from build123d import *

# Parameters (mm, degrees)
SKETCH1_W             = 156
SKETCH1_H             = 136
BOSS_EXTRUDE1_DEPTH   = 19.05
SKETCH2_W             = 37.5
SKETCH2_H             = 37.5
CUT_EXTRUDE1_DEPTH    = 106.218356288
SKETCH3_W             = 22.8
SKETCH3_H             = 12.5
CUT_EXTRUDE2_DEPTH    = 106.218356288
FILLET1_R             = 1
BOSS_EXTRUDE2_START   = -4.5
BOSS_EXTRUDE2_DEPTH   = 51.5
BOSS_EXTRUDE2_2_DEPTH = 3
BOSS_EXTRUDE2_START_2 = 44
BOSS_EXTRUDE2_3_DEPTH = 3
CUT_EXTRUDE3_REACH    = 130.365
SKETCH5_W             = 45.5
SKETCH5_H             = 6.35


# Read off the part's stored shape, not the designer's step: Boss-Extrude2
with BuildPart() as part:
    # Sketch1 → Boss-Extrude1 (new body)
    with BuildSketch(Plane(origin=(0, 0, 0), x_dir=(1, 0, 0), z_dir=(0, 1, 0))):
        Rectangle(SKETCH1_W, SKETCH1_H)
    extrude(amount=BOSS_EXTRUDE1_DEPTH)

    # Sketch2 → Cut-Extrude1 (cut, through all)
    with BuildSketch(Plane(origin=(0, 19.05, 0), x_dir=(1, 0, 0), z_dir=(0, 1, 0))):
        with Locations((32.5, -21.25)):
            Rectangle(SKETCH2_W, SKETCH2_H)
    extrude(amount=-CUT_EXTRUDE1_DEPTH, mode=Mode.SUBTRACT)

    # Sketch3 → Cut-Extrude2 (cut, through all)
    with BuildSketch(Plane(origin=(0, 19.05, 0), x_dir=(1, 0, 0), z_dir=(0, 1, 0))):
        with Locations((-32.65, -21.25)):
            Rectangle(SKETCH3_W, SKETCH3_H)
    extrude(amount=-CUT_EXTRUDE2_DEPTH, mode=Mode.SUBTRACT)

    # Fillet1
    fillet1_edges = [part.edges().sort_by_distance(p)[0] for p in [
        (-44.05, 19.05, 21.25),
        (-21.25, 19.05, 21.25),
    ]]
    fillet(fillet1_edges, radius=FILLET1_R)

    # Boss-Extrude2 outline → Boss-Extrude2 (add)
    with BuildSketch(Plane.XY.offset(BOSS_EXTRUDE2_START)):
        Polygon((-3, 19.05), (0, 19.05), (0, 73.655885813), (-3, 75.957866777), align=None)
    extrude(amount=BOSS_EXTRUDE2_DEPTH)

    # Boss-Extrude2 2 outline → Boss-Extrude2 2 (add)
    with BuildSketch(Plane.XY.offset(BOSS_EXTRUDE2_START)):
        Polygon((0, 73.655885813), (0, 19.05), (71.163775898, 19.05), align=None)
    extrude(amount=BOSS_EXTRUDE2_2_DEPTH)

    # Boss-Extrude2 3 outline → Boss-Extrude2 3 (add)
    with BuildSketch(Plane.XY.offset(BOSS_EXTRUDE2_START_2)):
        Polygon((0, 73.655885813), (0, 19.05), (71.163775898, 19.05), align=None)
    extrude(amount=BOSS_EXTRUDE2_3_DEPTH)

    # Sketch5 → Cut-Extrude3 (cut, up to next)
    with BuildSketch(Plane(origin=(0, 0, 0), x_dir=(0, 0, -1), z_dir=(1, 0, 0)), mode=Mode.PRIVATE) as cut_extrude3_sk1:
        with Locations((-21.25, 22.225)):
            Rectangle(SKETCH5_W, SKETCH5_H)
    cut_extrude3_tool1 = extrude(cut_extrude3_sk1.sketch, amount=-CUT_EXTRUDE3_REACH, mode=Mode.PRIVATE) & part.part
    add(cut_extrude3_tool1.solids().sort_by_distance((0, 22.225, 21.25))[0], mode=Mode.SUBTRACT)


solid = part.part
Input: part model. Units: mm. Frame: model coordinates. A direction names the side the tool comes from. Coordinates: 2 decimals unless noted, no trailing zeros. Loops run counter-clockwise (first coordinate to the right, second up) from the corner with the lowest first, then second, coordinate; pieces in that order, holes last. Notation, with made-up numbers: (-40, 44.25) -> (-14, 44.25) arc R19 ccw to (-14, 67.25) -> close; hole circle Ø4 at (41, 23). An arc over 180 degrees is marked (long way). One line per item, written item: value.
(1) Set-up query: faces 5 (the face through (-1, 9, 68)), 6 (the face through (17, 35, 47)), 7 (the face through (-3, 48, 21)), 8 (the face through (32, 10, 2.5)), 9 (the face through (17, 35, -4.5)). Return all of +Z, -Z, +X, -X, +Y, -Y with unobstructed straight access to the full face (end or side cutting, diameter ignored); none if empty.
Answer below:
face 5: +Z, +X, -X, +Y, -Y
face 6: +Z, +X, -X, +Y
face 7: +Z, -Z, -X, +Y
face 8: +Y, -Y
face 9: -Z, +X, -X, +Y
(2) Cut plane C-C (y = 7.5). Output: boundary loops of the cut face in (x, z), then the cut area to 3 significant figures.
Answer below:
outline: (-78, -68) -> (78, -68) -> (78, 68) -> (-78, 68) -> close; hole (-44.05, 15) -> (-21.25, 15) -> (-21.25, 27.5) -> (-44.05, 27.5) -> close; hole (13.75, 2.5) -> (51.25, 2.5) -> (51.25, 40) -> (13.75, 40) -> close
area: 19,500 mm2
(3) Ray query, line 1 along Z through (x, y) = (10.5, 63); line 2 along Y through (x, z) = (-57, 22.5); line 3 along Z through (x, y) = (-37.5, 18). Return the intervals inside material, ascending.
Answer below:
line 1: z = -4.5 to -1.5, 44 to 47
line 2: y = 0 to 19.05
line 3: z = -68 to 15, 27.5 to 68
(4) Cut plane D-D (x = -51.5). Output: boundary loops of the cut face in (y, z), then the cut area to 3 significant figures.
Answer below:
outline: (0, -68) -> (19.05, -68) -> (19.05, 68) -> (0, 68) -> close
area: 2,590 mm2
(5) Cut plane B-B (x = 48). Output: boundary loops of the cut face in (y, z), then the cut area to 3 significant figures.
Answer below:
outline: (0, -68) -> (19.05, -68) -> (19.05, -4.5) -> (36.82, -4.5) -> (36.82, -1.5) -> (19.05, -1.5) -> (19.05, 2.5) -> (0, 2.5) -> close; (0, 40) -> (19.05, 40) -> (19.05, 44) -> (36.82, 44) -> (36.82, 47) -> (19.05, 47) -> (19.05, 68) -> (0, 68) -> close
area: 1,980 mm2
(6) Draft query along X for faces 1 (the face through (25, 41, -1.5)), 2 (the face through (0, 49, 21)), 3 (the face through (13.75, 10, 22)), 4 (the face through (-33, 10, 15)). Return one class per face: pulls with the +X half, pulls with the -X half, needs draft (parallel to the pull), parting line crosses it, or undercut.
Answer below:
face 1: needs draft
face 2: pulls with the +X half
face 3: undercut
face 4: undercut
(7) Cut plane A-A (z = 19). Output: boundary loops of the cut face in (x, y), then the cut area to 3 significant figures.
Answer below:
outline: (-78, 0) -> (-44.05, 0) -> (-44.05, 18.05) arc R1 ccw to (-45.05, 19.05) -> (-78, 19.05) -> close; (-21.25, 0) -> (13.75, 0) -> (13.75, 19.05) -> (-20.25, 19.05) arc R1 ccw to (-21.25, 18.05) -> close; (-3, 25.4) -> (0, 25.4) -> (0, 73.66) -> (-3, 75.96) -> close; (51.25, 0) -> (78, 0) -> (78, 19.05) -> (51.25, 19.05) -> close
area: 1,970 mm2
(8) Pin query (flat end, axial travel): pin 1 Ø2 at (y, z) = (57, -1) entering from -X; pin 2 Ø1.5 at (y, z) = (25.5, 23) entering from +X; pin 3 Ø17 at (x, y) = (17, 45.5) entering from -Z. Return the tip coordinate at first contact, or that it passes through.
Answer below:
pin 1: stops at x = -3
pin 2: stops at x = 0
pin 3: stops at z = -4.5
